The listing builds one solid part. Answer for the finished solid, in the listing's coordinates (mm). A direction names the side the tool comes from. Round coordinates to 2 decimals unless told otherwise and drop trailing zeros. Write each loop counter-clockwise with the first axis right and the second up, starting at its lowest first coordinate (ties: lowest second). Pieces come first, ordered by that corner, then holes.
Item 1: Find the intervals of material crossed by probe 1 along Z at (x, y) = (7, 4); probe 2 along Z at (x, y) = (10.5, 7); probe 3 along X at (y, z) = (0.5, 13), in increasing order.
Item 2: Find section C-C on z = 13. Give the vertices of the cut face in (x, y), then the cut area to 3 significant figures.
Item 3: A tool of negligible diameter and unlimited length cuts with its end or side. For faces 4 (the face through (20, 4, 9)), 5 (the face through (7.605, 1.699, 14.765)), 6 (the face through (7, 4, 3)), from which of +Z, -Z, +X, -X, +Y, -Y can it reach the whole face along a straight path? Write none if from no direction.
Item 4: For a pull along Z with two mould halves and no side action, classify faces 1 (the face through (17, 8, 5)), 2 (the face through (15, 4, 9)), 3 (the face through (10, 4, 0)) as +Z half, -Z half, draft (parallel to the pull), parting line (faces both ways), or undercut.
Item 5: Find section D-D on y = 5. Give the vertices of the cut face in (x, z), then the cut area to 3 significant figures.
Item 6: Each of these flat-tipped pins is pushed along its axis until it touches: pin 1 (2 mm diameter, centred on x = 9.5, y = 6, fed in from -Z); pin 2 (3 mm diameter, centred on x = 2, y = 7, fed in from +Z). Where does it stop, or does it pass through?
Item 7: Find section A-A on x = 13.75. Give the vertices of the cut face in (y, z), then the cut area to 3 significant figures.
Item 8: Find section B-B on y = 4. Give the vertices of the cut face in (x, z), then the cut area to 3 significant figures.
```python
from build123d import *

# Parameters (mm, degrees)
ESQUISSE1_W        = 20
ESQUISSE1_H        = 8
BOSS_EXTRU_1_DEPTH = 3
ESQUISSE2_W        = 5
ESQUISSE2_H        = 8
BOSS_EXTRU_2_DEPTH = 15
ESQUISSE3_R        = 2.9
BOSS_EXTRU_3_DEPTH = 15


with BuildPart() as part:
    # Esquisse1 → Boss.-Extru.1 (new body)
    with BuildSketch(Plane.XY):
        with Locations((10, 4)):
            Rectangle(ESQUISSE1_W, ESQUISSE1_H)
    extrude(amount=BOSS_EXTRU_1_DEPTH)

    # Esquisse2 → Boss.-Extru.2 (add)
    with BuildSketch(Plane.XY.offset(3)):
        with Locations((17.5, 4)):
            Rectangle(ESQUISSE2_W, ESQUISSE2_H)
    extrude(amount=BOSS_EXTRU_2_DEPTH)

    # Esquisse3 → Boss.-Extru.3 (add)
    with BuildSketch(Plane.ZY.offset(-15)):
        with Locations(Location((13, 4, 0), (0, 0, 90))):
            Circle(ESQUISSE3_R)
    extrude(amount=BOSS_EXTRU_3_DEPTH)


solid = part.part
```
Check values:
1. probe 1: z = 0 to 3, 10.1 to 15.9
1. probe 2: z = 0 to 3
1. probe 3: x = 15 to 20
2. outline: (0, 1.1) - (15, 1.1) - (15, 0) - (20, 0) - (20, 8) - (15, 8) - (15, 6.9) - (0, 6.9) - close
2. area: 127 mm2
3. face 4: +Z, -Z, +X, +Y, -Y
3. face 5: -X
3. face 6: -X, +Y, -Y
4. face 1: draft
4. face 2: undercut
4. face 3: -Z half
5. outline: (0, 0) - (20, 0) - (20, 18) - (15, 18) - (15, 15.72) - (0, 15.72) - (0, 10.28) - (15, 10.28) - (15, 3) - (0, 3) - close
5. area: 217 mm2
6. pin 1: stops at z = 0
6. pin 2: stops at z = 15.48
7. outline: (0, 0) - (8, 0) - (8, 3) - (0, 3) - close; circle Ø5.8 at (4, 13)
7. area: 50.4 mm2
8. outline: (0, 0) - (20, 0) - (20, 18) - (15, 18) - (15, 15.9) - (0, 15.9) - (0, 10.1) - (15, 10.1) - (15, 3) - (0, 3) - close
8. area: 222 mm2
